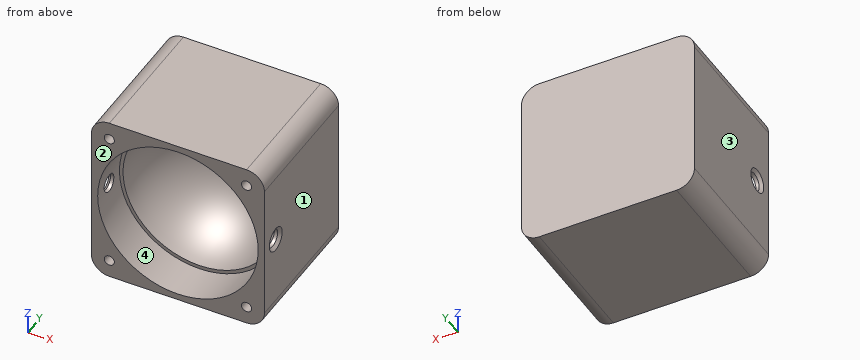
```python
from build123d import *

# Parameters (mm, degrees)
SKETCH1_W           = 29
SKETCH1_H           = 29
BOSS_EXTRUDE1_DEPTH = 23
FILLET1_R           = 3
SKETCH2_R           = 13.45
CUT_EXTRUDE1_DEPTH  = 6.75
SKETCH7_R           = 0.85
CUT_EXTRUDE2_DEPTH  = 10
SKETCH8_R           = 1.5
CUT_EXTRUDE3_DEPTH  = 30
CHAMFER1_SIZE       = 0.5


with BuildPart() as part:
    # Sketch1 → Boss-Extrude1 (new body)
    with BuildSketch(Plane(origin=(0, 0, 0), x_dir=(1, 0, 0), z_dir=(0, 1, 0))):
        with Locations((14.5, 14.5)):
            Rectangle(SKETCH1_W, SKETCH1_H)
    extrude(amount=BOSS_EXTRUDE1_DEPTH)

    # Fillet1
    fillet1_edges = [part.edges().sort_by_distance(p)[0] for p in [
        (0, 11.5, -29),
        (29, 11.5, -29),
        (29, 11.5, 0),
        (0, 11.5, 0),
    ]]
    fillet(fillet1_edges, radius=FILLET1_R)

    # Sketch2 → Cut-Extrude1 (cut)
    with BuildSketch(Plane.XZ):
        with Locations((14.5, -14.5)):
            Circle(SKETCH2_R)
    extrude(amount=-CUT_EXTRUDE1_DEPTH, mode=Mode.SUBTRACT)

    # Sketch6 → Cut-Revolve1 (revolve, cut)
    with BuildSketch(Plane(origin=(14.5, 0, 0), x_dir=(0, 0, -1), z_dir=(1, 0, 0))):
        with BuildLine():
            Line((14.5, 6.75), (14.5, 19.6))
            ThreePointArc((14.5, 19.6), (23.586322138, 15.836322138), (27.35, 6.75))
            Line((27.35, 6.75), (14.5, 6.75))
        make_face()
    revolve(axis=Axis((14.5, 6.75, -14.5), (0, 1, 0)), mode=Mode.SUBTRACT)

    # Sketch7 → Cut-Extrude2 (cut)
    with BuildSketch(Plane.XZ):
        with Locations((3, -3)):
            Circle(SKETCH7_R)
        with Locations((26, -3)):
            Circle(SKETCH7_R)
        with Locations((26, -26)):
            Circle(SKETCH7_R)
        with Locations((3, -26)):
            Circle(SKETCH7_R)
    extrude(amount=-CUT_EXTRUDE2_DEPTH, mode=Mode.SUBTRACT)

    # Sketch8 → Cut-Extrude3 (cut, through all)
    with BuildSketch(Plane.ZY):
        with Locations((-14.5, 3.5)):
            Circle(SKETCH8_R)
    extrude(amount=-CUT_EXTRUDE3_DEPTH, mode=Mode.SUBTRACT)

    # Chamfer1
    chamfer1_edges = [part.edges().sort_by_distance(p)[0] for p in [
        (29, 3.5, -16),
        (0, 3.5, -16),
    ]]
    chamfer(chamfer1_edges, length=CHAMFER1_SIZE)


solid = part.part
```
Part model, mm, in its own coordinate system. Face numbers are marked on the shaded views. Give positions to 0.01 mm unless a question says otherwise; leave off trailing zeros. Order: outer loops, then holes, each group sorted by start corner. A loop starts at its lowest first (then second) coordinate and runs counter-clockwise, first axis right, second up. Notation, with made-up numbers: (6.25, 35) - (25.25, 35) arc R30 ccw to (25.25, 63) - close; hole circle Ø3 at (-15, -26). An arc over 180 degrees is marked (long way). Use one line per item in the form item = value.
Item 1: Slice it at A-A on y = 3.5. Give the cut face in (x, z), and give its area (3 significant figures).
Solution:
outline = (0, -26) arc R3 ccw to (3, -29) - (26, -29) arc R3 ccw to (29, -26) - (29, -16.5) - (28.5, -16) - (27.87, -16) arc R13.45 cw to (1.13, -16) - (0.5, -16) - (0, -16.5) - close; (0, -12.5) - (0.5, -13) - (1.13, -13) arc R13.45 cw to (27.87, -13) - (28.5, -13) - (29, -12.5) - (29, -3) arc R3 ccw to (26, 0) - (3, 0) arc R3 ccw to (0, -3) - close; hole circle Ø1.7 at (3, -26); hole circle Ø1.7 at (3, -3); hole circle Ø1.7 at (26, -26); hole circle Ø1.7 at (26, -3)
area = 249 mm2
Item 2: Slice it at C-C on x = 23. Give the cut face in (y, z), and give its area (3 significant figures).
Solution:
outline = (0, -29) - (23, -29) - (23, 0) - (0, 0) - (0, -4.08) - (6.75, -4.08) - (6.75, -4.86) arc R9.64 cw to (6.75, -24.14) - (6.75, -24.92) - (0, -24.92) - close
area = 380 mm2
Item 3: Probe probe 1 along X at (y, z) = (6, -15); probe 2 along Y at (x, z) = (28.2, -14.5); probe 3 along X at (y, z) = (1.75, -25.75). List the from-to ranges inside material, lowest first. Write a range as from..to.
Solution:
probe_1 = 0..1.06, 27.94..29
probe_2 = 0..2, 5..23
probe_3 = 0..2.19, 3.81..7.13, 21.87..25.19, 26.81..29
Item 4: Slice it at D-D on z = -9.5. Give the cut face in (x, y).
Solution:
outline = (0, 0) - (2.01, 0) - (2.01, 6.75) - (2.66, 6.75) arc R11.84 cw to (26.34, 6.75) - (26.99, 6.75) - (26.99, 0) - (29, 0) - (29, 23) - (0, 23) - close
Item 5: Two-plate mould, pull along X, no slides. Class the marked faces 1, 2, 3 and 4: released by +X, released by -X, zero draft, split by the parting line, or undercut.
Solution:
face_1 = released by +X
face_2 = zero draft
face_3 = released by -X
face_4 = undercut
Item 6: Pin check, flat tips, straight feed: pin 1 Ø1.9 at (x, z) = (26, -26) entering from -Y; pin 2 Ø8 at (x, z) = (10.5, -10) entering from -Y. Stop position of each tip, or through.
Solution:
pin_1 = 0
pin_2 = 14.79
Item 7: Slice it at B-B on z = -14.5. Give the cut face in (x, y).
Solution:
outline = (0, 0) - (1.05, 0) - (1.05, 2) - (0.5, 2) - (0, 1.5) - close; (0, 5.5) - (0.5, 5) - (1.05, 5) - (1.05, 6.75) - (1.65, 6.75) arc R12.85 cw to (27.35, 6.75) - (27.95, 6.75) - (27.95, 5) - (28.5, 5) - (29, 5.5) - (29, 23) - (0, 23) - close; (27.95, 0) - (29, 0) - (29, 1.5) - (28.5, 2) - (27.95, 2) - close
